Here's how the part is built. I have some questions about the finished solid (model axes, mm). Face numbers are marked on the shaded views. Give positions to 0.01 mm unless a question says otherwise; leave off trailing zeros. Loops run counter-clockwise (first coordinate to the right, second up) from the corner with the lowest first, then second, coordinate; pieces in that order, holes last. Notation, with made-up numbers: (78.25, 40) - (110.25, 40) arc R9 ccw to (110.25, 50) - close; hole circle Ø3 at (25, 54.5). An arc over 180 degrees is marked (long way). Return JSON: item names as keys, results as strings. Group by question number.
(1) I need wall thicknesses on probe 1 along Z at (x, y) = (61, -62.5); probe 2 along Y at (x, z) = (-6.5, 49); probe 3 along Y at (x, z) = (-48, 53). Which ranges of each line are inside material? Lowest first, please. Write a range as [from, to].
(2) If we section it at A-A (z = 57): Please give me the cut outline in (x, y).
(3) If we section it at C-C (y = -15.5): Please give me the cut outline in (x, z).
(4) For P1, Ø6.5, axis at x = -41.5, y = -34, coming from the +Z side, with a flat end and sliding along its axis, tell me the tip position at first contact or that it passes through.
(5) If we section it at D-D (y = -34.5): Please give me the cut outline in (x, z).
(6) If we section it at B-B (x = -4.5): Please give me the cut outline in (y, z).
(7) If we mould it in two halves opening along Y, with no side actions, what happens to the marked faces 1, 2 and 3? For each: released by +Y, released by -Y, zero draft, split by the parting line, or undercut.
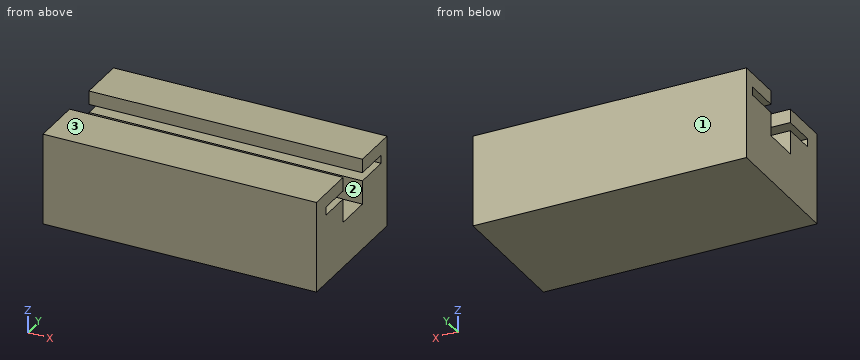
```python
from build123d import *

# Parameters (mm, degrees)
F0_W     = 152.4
F0_H     = 50.8
F1_DEPTH = 76.2
F2_W     = 59.863596
F2_H     = 4.604891
F3_DEPTH = 152.4
F4_W     = 152.4
F4_H     = 20.887783
F5_DEPTH = 25.4


with BuildPart() as f1:
    # F0 (on Front) → F1 (new body)
    with BuildSketch(Plane.XZ):
        with Locations((-4.536367, 36.624424)):
            Rectangle(F0_W, F0_H)
    extrude(amount=F1_DEPTH)

    # F2 (on face) → F3 (cut, through all)
    with BuildSketch(Plane.YZ.offset(71.663633)):
        with Locations((-36.263526, 52.092843)):
            Rectangle(F2_W, F2_H)
    extrude(amount=-F3_DEPTH, mode=Mode.SUBTRACT)

    # F4 (on face) → F5 (cut)
    with BuildSketch(Plane.XY.offset(62.024424)):
        with Locations((-4.536367, -36.993027)):
            Rectangle(F4_W, F4_H)
    extrude(amount=-F5_DEPTH, mode=Mode.SUBTRACT)


solid = f1.part
```
Values:
{
 "1": {"probe 1": "[11.22, 49.79], [54.4, 62.02]", "probe 2": "[-76.2, -47.44], [-26.55, 0]", "probe 3": "[-76.2, -66.2], [-6.33, 0]"},
 "2": {"outline": "(-80.74, -76.2) - (71.66, -76.2) - (71.66, -47.44) - (-80.74, -47.44) - close; (-80.74, -26.55) - (71.66, -26.55) - (71.66, 0) - (-80.74, 0) - close"},
 "3": {"outline": "(-80.74, 11.22) - (71.66, 11.22) - (71.66, 49.79) - (-80.74, 49.79) - close; (-80.74, 54.4) - (71.66, 54.4) - (71.66, 62.02) - (-80.74, 62.02) - close"},
 "4": {"P1": "z = 36.62"},
 "5": {"outline": "(-80.74, 11.22) - (71.66, 11.22) - (71.66, 36.62) - (-80.74, 36.62) - close"},
 "6": {"outline": "(-76.2, 11.22) - (0, 11.22) - (0, 62.02) - (-26.55, 62.02) - (-26.55, 54.4) - (-6.33, 54.4) - (-6.33, 49.79) - (-26.55, 49.79) - (-26.55, 36.62) - (-47.44, 36.62) - (-47.44, 49.79) - (-66.2, 49.79) - (-66.2, 54.4) - (-47.44, 54.4) - (-47.44, 62.02) - (-76.2, 62.02) - close"},
 "7": {"face 1": "released by +Y", "face 2": "undercut", "face 3": "zero draft"}
}
